Print and shaded views of the part. All mm, measured from the part's lowest x, y and z. A direction names the side the tool comes from. Coordinates: 2 decimals unless noted, no trailing zeros. Return JSON: item names as keys, results as strings. Group by question number.
1) Flat gauge pins, fed straight in: pin 1 (12 mm diameter, centred on x = 13, y = 30.5, fed in from +Z); pin 2 (5 mm diameter, centred on x = 30, z = 148.5, fed in from -Y); pin 3 (10 mm diameter, centred on y = 25.5, z = 12.5, fed in from +X); pin 4 (3 mm diameter, centred on x = 21, y = 11, fed in from -Z). Where does each tip first touch, or does it go through?
2) Probe line 1 (Z direction, x = 15.5, y = 30); line 2 (Z direction, x = 11, y = 30); line 3 (Z direction, x = 23, y = 17). List the from-to ranges inside material, lowest first.
3) Which spindle directions (+Z, -Z, +X, -X, +Y, -Y) get a long thin tool onto all of the face, cutting with end or side? Do the marked faces 1, 2, 3 and 4. Say none if no direction does.
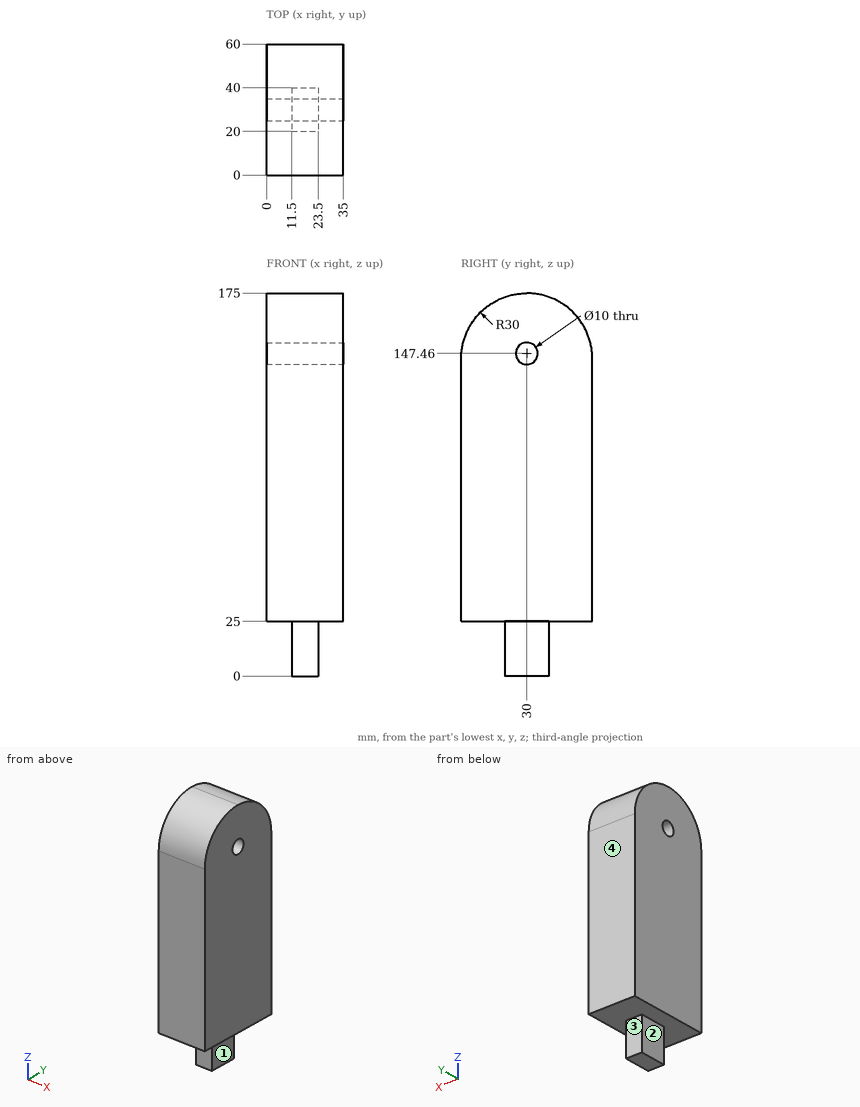
Answers below:
{
 "1": {"pin 1": "stops at z = 175", "pin 2": "stops at y = 0.02", "pin 3": "stops at x = 23.5", "pin 4": "stops at z = 25"},
 "2": {"line 1": "z = 0 to 142.46, 152.46 to 175", "line 2": "z = 25 to 142.46, 152.46 to 175", "line 3": "z = 25 to 172.04"},
 "3": {"face 1": "-Z, +X, +Y, -Y", "face 2": "-Z, -X, +Y, -Y", "face 3": "-Z, +X, -X, +Y", "face 4": "+Z, -Z, +X, -X, +Y"}
}
